Read the model definition and answer for the solid it produces. Units are mm, in the model's axes. Give positions to 0.01 mm unless a question says otherwise; leave off trailing zeros. Loops run counter-clockwise (first coordinate to the right, second up) from the corner with the lowest first, then second, coordinate; pieces in that order, holes last. Notation, with made-up numbers: (-12.5, 13) - (-7.5, 13) arc R26 ccw to (-7.5, 37) - close; hole circle Ø9 at (-27, 10.25). An arc over 180 degrees is marked (long way). Use a Markdown table: item, result. Add a question column.
Item 1: Consider probe 1 along X at (y, z) = (330.5, 0.65); probe 2 along X at (y, z) = (93.5, 0.1). Determine where each line is inside the solid, lowest interval first. Write a range as [from, to].
Item 2: A cutting plane is placed at B-B (x = 150). Determine the outline of the cut face in (y, z), plus the area to 3 significant figures.
Item 3: A cutting plane is placed at A-A (z = 0.6). Determine the outline of the cut face in (x, y).
Item 4: Each of these flat-tipped pins is pushed along its axis until it touches: P1, Ø0.5, axis at x = 154.5, z = 0.5, coming from the +Y side; P2, Ø0.5, axis at y = 250.5, z = 0.5, coming from the +X side; P3, Ø0.5, axis at y = 214, z = 0.5, coming from the -X side. Where does it stop, or does it pass through?
from build123d import *

# Parameters (mm, degrees)
F1_DEPTH = 1


with BuildPart() as f1:
    # F0 (on Top) → F1 (new body)
    with BuildSketch(Plane.XY):
        with BuildLine():
            ThreePointArc((-16, 125.988095), (-89.802561, 89.802561), (-125.988095, 16))
            Line((-125.988095, 16), (-190, 16))
            Line((-190, 16), (-190, 0))
            Line((-190, 0), (-190, -16))
            Line((-190, -16), (-16, -16))
            Line((-16, -16), (-16, -133.589491))
            Line((-16, -133.589491), (0, -133.589491))
            Line((0, -133.589491), (16, -133.589491))
            Line((16, -133.589491), (16, -16))
            Line((16, -16), (190, -16))
            Line((190, -16), (190, 0))
            Line((190, 0), (190, 16))
            Line((190, 16), (125.988095, 16))
            ThreePointArc((125.988095, 16), (89.802561, 89.802561), (16, 125.988095))
            Line((16, 125.988095), (16, 371.410509))
            Line((16, 371.410509), (0, 371.410509))
            Line((0, 371.410509), (-16, 371.410509))
            Line((-16, 371.410509), (-16, 125.988095))
        make_face()
    extrude(amount=F1_DEPTH)


solid = f1.part
Geometry says:
| question | item | result |
|---|---|---|
| 1 | probe 1 | [-16, 16] |
| 1 | probe 2 | [-85.95, 85.95] |
| 2 | outline | (-16, 0) - (16, 0) - (16, 1) - (-16, 1) - close |
| 2 | area | 32.0 mm² |
| 3 | outline | (-190, -16) - (-16, -16) - (-16, -133.59) - (16, -133.59) - (16, -16) - (190, -16) - (190, 16) - (125.99, 16) arc R127 ccw to (16, 125.99) - (16, 371.41) - (-16, 371.41) - (-16, 125.99) arc R127 ccw to (-125.99, 16) - (-190, 16) - close |
| 4 | P1 | y = 16 |
| 4 | P2 | x = 16 |
| 4 | P3 | x = -16 |
